Could you check a few things on this model? Use its own coordinates, in mm. Face numbers are marked on the shaded views. A direction names the side the tool comes from. Give positions to 0.01 mm unless a question says otherwise; leave off trailing zeros. Loops run counter-clockwise (first coordinate to the right, second up) from the corner with the lowest first, then second, coordinate; pieces in that order, holes last. Notation, with made-up numbers: M 55,-30.5 L 103,-30.5 A18 ccw 103,2.5 Z; hole C 49.5,80 d3. An arc over 180 degrees is marked long. Return JSON: item names as keys, results as strings. Group by question number.
1. If we section it at C-C (z = -1): Write out the boundary of the cut face in (x, y).
2. If we section it at A-A (x = -4.5): Write out the boundary of the cut face in (y, z), plus the area to 3 significant figures.
3. If we section it at D-D (y = -3.5): Write out the boundary of the cut face in (x, z).
4. If we section it at B-B (y = -1.25): Write out the boundary of the cut face in (x, z), plus the area to 3 significant figures.
5. For the marked faces 5 and 6, which set-ups out of +Z, -Z, +X, -X, +Y, -Y let a thin tool reach every point of the face, with its end or its side?
6. If we mould it in two halves opening along X, with no side actions, what happens to the marked faces 1, 2, 3 and 4? For each: +X half, -X half, draft (parallel to the pull), parting line (faces both ways), or undercut.
7. Please list where these lines run through material, in increasing order: line 1 (X direction, y = 1.75, z = 2.25); line 2 (Y direction, x = 5.5, z = -0.95); line 3 (Y direction, x = -9.5, z = -2).
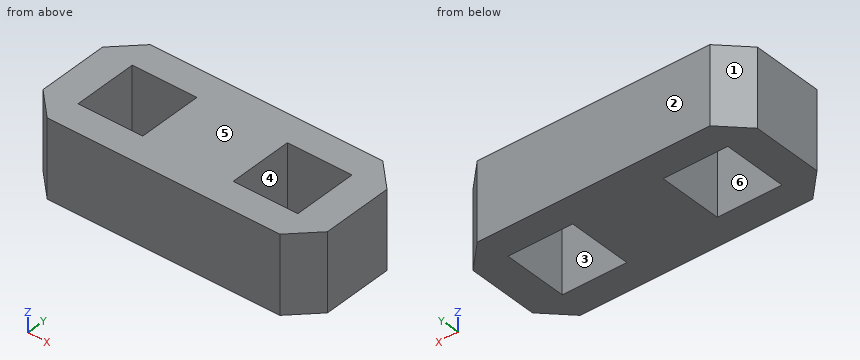
```python
from build123d import *

# Parameters (mm, degrees)
SKETCH_1_W          = 22
SKETCH_1_H          = 9.5
EXTRUDE_1_DEPTH     = 3
SKETCH_2_W          = 5
SKETCH_2_H          = 5
CUT_EXTRUDE_1_DEPTH = 14.400093283
CHAMFER_1_SIZE      = 2


with BuildPart() as part:
    # 草图1 → 凸台-拉伸1 (new, symmetric)
    with BuildSketch(Plane.XY):
        Rectangle(SKETCH_1_W, SKETCH_1_H)
    extrude(amount=EXTRUDE_1_DEPTH, both=True)

    # 草图2 → 切除-拉伸1 (cut, through all)
    with BuildSketch(Plane.XY.offset(3)):
        with Locations((6, 0)):
            Rectangle(SKETCH_2_W, SKETCH_2_H)
    cut_extrude_1 = extrude(amount=-CUT_EXTRUDE_1_DEPTH, mode=Mode.SUBTRACT)

    # 镜向1: 切除-拉伸1 across plane
    add(cut_extrude_1.mirror(Plane(origin=(0, 0, 0), x_dir=(0, 0, 1), z_dir=(1, 0, 0))), mode=Mode.SUBTRACT)

    # 倒角1
    chamfer_1_edges = [part.edges().sort_by_distance(p)[0] for p in [
        (11, -4.75, 0),
        (-11, -4.75, 0),
        (-11, 4.75, 0),
        (11, 4.75, 0),
    ]]
    chamfer(chamfer_1_edges, length=CHAMFER_1_SIZE)


solid = part.part
```
Answer:
{
 "1": {"outline": "M -11,-2.75 L -9,-4.75 L 9,-4.75 L 11,-2.75 L 11,2.75 L 9,4.75 L -9,4.75 L -11,2.75 Z; hole M -8.5,-2.5 L -3.5,-2.5 L -3.5,2.5 L -8.5,2.5 Z; hole M 3.5,-2.5 L 8.5,-2.5 L 8.5,2.5 L 3.5,2.5 Z"},
 "2": {"outline": "M -4.75,-3 L -2.5,-3 L -2.5,3 L -4.75,3 Z; M 2.5,-3 L 4.75,-3 L 4.75,3 L 2.5,3 Z", "area": "27.0 mm²"},
 "3": {"outline": "M -10.25,-3 L 10.25,-3 L 10.25,3 L -10.25,3 Z"},
 "4": {"outline": "M -11,-3 L -8.5,-3 L -8.5,3 L -11,3 Z; M -3.5,-3 L 3.5,-3 L 3.5,3 L -3.5,3 Z; M 8.5,-3 L 11,-3 L 11,3 L 8.5,3 Z", "area": "72.0 mm²"},
 "5": {"face 5": "+Z, +X, -X, +Y, -Y", "face 6": "+Z, -Z"},
 "6": {"face 1": "-X half", "face 2": "draft", "face 3": "undercut", "face 4": "undercut"},
 "7": {"line 1": "x = -11 to -8.5, -3.5 to 3.5, 8.5 to 11", "line 2": "y = -4.75 to -2.5, 2.5 to 4.75", "line 3": "y = -4.25 to 4.25"}
}
